Work out the finished part from the listing and answer in its coordinate system (mm). A direction names the side the tool comes from. Coordinates: 2 decimals unless noted, no trailing zeros. Write each loop counter-clockwise with the first axis right and the second up, starting at its lowest first coordinate (ties: lowest second). Pieces come first, ordered by that corner, then holes. Notation, with made-up numbers: (89, 56.5) - (135, 56.5) arc R14 cw to (135, 71.5) - close; hole circle Ø5 at (68.25, 44). An arc over 180 degrees is marked (long way). Answer as a JSON object with one key per item and string values. Group by question number.
from build123d import *

# Parameters (mm, degrees)
EXTRUDE_1_DEPTH     = 17.5
SKETCH_2_R          = 4
CUT_EXTRUDE_1_DEPTH = 44.283946216
SKETCH_3_W          = 29
SKETCH_3_H          = 25.5
CUT_EXTRUDE_2_DEPTH = 44.686382318
CUT_EXTRUDE_3_REACH = 40.22
SKETCH_4_R          = 5.3
FILLET_1_R          = 1
FILLET_2_R          = 2


with BuildPart() as part:
    # ｽｹｯﾁ1 → ﾎﾞｽ - 押し出し1 (new, symmetric)
    with BuildSketch(Plane.XY):
        with BuildLine():
            Line((-18.5, 11), (-18.5, -13))
            Line((-18.5, -13), (-11.715374514, -13))
            ThreePointArc((-11.715374514, -13), (12.037359531, -12.702439747), (13.610657589, 11))
            Line((13.610657589, 11), (-18.5, 11))
        make_face()
    extrude(amount=EXTRUDE_1_DEPTH, both=True)

    # ｽｹｯﾁ2 → ｶｯﾄ - 押し出し1 (cut, through all)
    with BuildSketch(Plane.XY.offset(17.5)):
        Circle(SKETCH_2_R)
        with BuildLine():
            Line((-18.5, 2), (-11.5, 2))
            ThreePointArc((-11.5, 2), (-7.5, -2), (-11.5, -6))
            Line((-11.5, -6), (-18.5, -6))
            Line((-18.5, -6), (-18.5, 2))
        make_face()
    extrude(amount=-CUT_EXTRUDE_1_DEPTH, mode=Mode.SUBTRACT)

    # ｽｹｯﾁ3 → ｶｯﾄ - 押し出し2 (cut, through all)
    with BuildSketch(Plane.ZY.offset(18.5)):
        with Locations((0, -4.75)):
            Rectangle(SKETCH_3_W, SKETCH_3_H)
    extrude(amount=-CUT_EXTRUDE_2_DEPTH, mode=Mode.SUBTRACT)

    # ｽｹｯﾁ4 → ｶｯﾄ - 押し出し3 (cut, up to next)
    with BuildSketch(Plane(origin=(0, 11, 0), x_dir=(1, 0, 0), z_dir=(0, 1, 0)), mode=Mode.PRIVATE) as cut_extrude_3_sk1:
        with Locations(Location((0.610657589, 0, 0), (0, 0, 270))):
            Circle(SKETCH_4_R)
    cut_extrude_3_tool1 = extrude(cut_extrude_3_sk1.sketch, amount=-CUT_EXTRUDE_3_REACH, mode=Mode.PRIVATE) & part.part
    add(cut_extrude_3_tool1.solids().sort_by_distance((0.610658, 11, 0))[0], mode=Mode.SUBTRACT)

    # ﾌｨﾚｯﾄ1
    fillet_1_edges = [part.edges().sort_by_distance(p)[0] for p in [
        (-18.5, -6, -16),
        (-18.5, 2, -16),
        (-18.5, -6, 16),
        (-18.5, 2, 16),
        (-18.5, -13, -16),
        (-18.5, -13, 16),
    ]]
    fillet(fillet_1_edges, radius=FILLET_1_R)

    # ﾌｨﾚｯﾄ2
    fillet_2_edges = [part.edges().sort_by_distance(p)[0] for p in [
        (-2.444671206, 11, 17.5),
        (-1.467808792, 8, -14.5),
        (-1.467808792, 8, 14.5),
        (-2.444671206, 11, -17.5),
    ]]
    fillet(fillet_2_edges, radius=FILLET_2_R)


solid = part.part
Q1. Consider L1, parallel to Y at x = 0, z = 15; L2, parallel to Z at x = -2, y = -15.5; L3, parallel to Y at x = -15.5, z = -5.5. Determine where each line is inside the solid, lowest interval first. Write a range as from..to.
Q2. For a pull along Z with two mould halves and no side action, classify faces 1 (the face through (-18.5, -9, -16)), 2 (the face through (-2.61, 9.52, -4.21)) as +Z half, -Z half, draft (parallel to the pull), parting line (faces both ways), or undercut.
Q3. Section A-A on y = -10.5 is taken. Determine the outline of the cut face in (x, z), plus the area to 3 significant figures.
Q4. Section C-C on x = 2 is taken. Determine the outline of the cut face in (y, z).
Q5. Flat-ended cylindrical pins translate along their axes: pin 1 Ø12 at (x, z) = (0.61, 0) entering from -Y; pin 2 Ø2.5 at (x, z) = (-13.5, 16.5) entering from -Y; pin 3 Ø2.5 at (x, z) = (-15.5, -16.5) entering from +Y; pin 4 Ø0.9 at (x, z) = (-15, 16.5) entering from +Y. Find the tip coordinate at first contact, or state that the pin passes through.
Q6. A tool of negligible diameter and unlimited length cuts with its end or side. For faces 3 (the face through (-0.79, 7.4, 13.93)), 4 (the face through (-6, 11, 0)), 5 (the face through (-15, -13, 16)), 6 (the face through (-18.215, 2.301, 15.979)), from which of +Z, -Z, +X, -X, +Y, -Y can it reach the whole face along a straight path? Write none if from no direction.
Q7. Section D-D on y = -1.75 is taken. Determine the outline of the cut face in (x, z).
Q8. Section B-B on z = 0 is taken. Determine the outline of the cut face in (x, y).
Numbers:
{
 "1": {"L1": "y = -17.5..-4, 4..11", "L2": "z = -17.5..-14.5, 14.5..17.5", "L3": "y = 8..11"},
 "2": {"face 1": "draft", "face 2": "undercut"},
 "3": {"outline": "(-18.5, -17.5) - (14, -17.5) - (14, -14.5) - (-18.5, -14.5) - close; (-18.5, 14.5) - (14, 14.5) - (14, 17.5) - (-18.5, 17.5) - close", "area": "195 mm²"},
 "4": {"outline": "(-17.39, -17.5) - (-3.46, -17.5) - (-3.46, -14.5) - (-17.39, -14.5) - close; (-17.39, 14.5) - (-3.46, 14.5) - (-3.46, 17.5) - (-17.39, 17.5) - close; (3.46, -17.5) - (9, -17.5) arc R2 ccw to (11, -15.5) - (11, -5.11) - (8, -5.11) - (8, -12.5) arc R2 cw to (6, -14.5) - (3.46, -14.5) - close; (3.46, 14.5) - (6, 14.5) arc R2 cw to (8, 12.5) - (8, 5.11) - (11, 5.11) - (11, 15.5) arc R2 ccw to (9, 17.5) - (3.46, 17.5) - close"},
 "5": {"pin 1": "stops at y = 8", "pin 2": "stops at y = -13", "pin 3": "stops at y = 11", "pin 4": "stops at y = 10.92"},
 "6": {"face 3": "+X, -X, -Y", "face 4": "+Z, -Z, +X, -X, +Y", "face 5": "+Z, -Z, -X, -Y", "face 6": "+Z, -Z, -X"},
 "7": {"outline": "(-7.51, -17.5) - (-3.6, -17.5) - (-3.6, -14.5) - (-7.51, -14.5) - close; (-7.51, 14.5) - (-3.6, 14.5) - (-3.6, 17.5) - (-7.51, 17.5) - close; (3.6, -17.5) - (17.41, -17.5) - (17.41, -14.5) - (3.6, -14.5) - close; (3.6, 14.5) - (17.41, 14.5) - (17.41, 17.5) - (3.6, 17.5) - close"},
 "8": {"outline": "(-18.5, 8) - (-4.69, 8) - (-4.69, 11) - (-18.5, 11) - close; (5.91, 8) - (15.56, 8) arc R17.5 ccw to (13.61, 11) - (5.91, 11) - close"}
}
